from build123d import *

# Parameters (mm, degrees)
F3_DEPTH = 12.7
F5_DEPTH = 12.7


with BuildPart() as f1:
    # F0 (on Front) → F1 (revolve)
    with BuildSketch(Plane.XZ):
        with BuildLine():
            ThreePointArc((17.4752, 17.537158), (8.874046, 19.85641), (0, 20.6375))
            ThreePointArc((0, 20.6375), (-8.874046, 19.85641), (-17.4752, 17.537158))
            Line((-17.4752, 17.537158), (-17.4752, 0))
            Line((-17.4752, 0), (17.4752, 0))
            Line((17.4752, 0), (17.4752, 17.537158))
        make_face()
    revolve(axis=Axis((-4.40496, 0, 0), (1, 0, 0)))

    # F2 (on face) → F3 (cut)
    with BuildSketch(Plane.YZ.offset(17.4752)):
        Polygon((4.7879, -2.764295), (4.7879, 2.764295), (0, 5.528591), (-4.7879, 2.764295), (-4.7879, -2.764295), (0, -5.528591), align=None)
    extrude(amount=-F3_DEPTH, mode=Mode.SUBTRACT)

    # F4 (on face) → F5 (join)
    with BuildSketch(Plane(origin=(-17.4752, 0, 0), x_dir=(0, -1, 0), z_dir=(-1, 0, 0))):
        Polygon((4.7625, -2.749631), (4.7625, 2.749631), (0, 5.499261), (-4.7625, 2.749631), (-4.7625, -2.749631), (0, -5.499261), align=None)
    extrude(amount=F5_DEPTH)


solid = f1.part
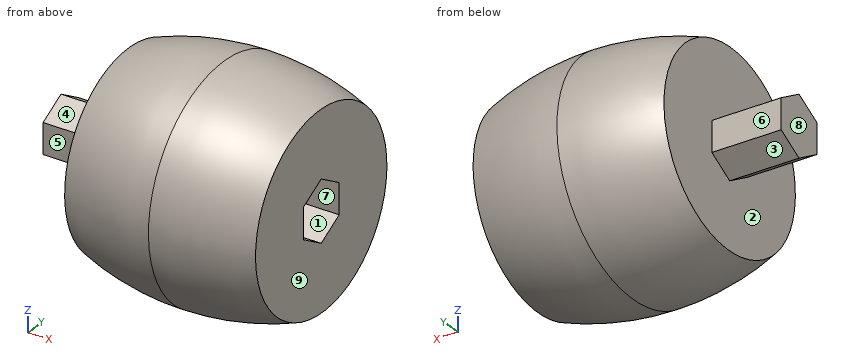
Verification items for the finished model (mm, model axes). Face numbers are marked on the shaded views. A direction names the side the tool comes from. Round coordinates to 2 decimals unless told otherwise and drop trailing zeros. Loops run counter-clockwise (first coordinate to the right, second up) from the corner with the lowest first, then second, coordinate; pieces in that order, holes last. Notation, with made-up numbers: (89.25, -34.75) - (126.25, -34.75) arc R18 ccw to (126.25, -17.75) - close; hole circle Ø10 at (-12.75, -38.75). An arc over 180 degrees is marked (long way). Use a Markdown table: item, result. Add a question column.
1. Gauge pin test, flat ends, axial feed: pin 1 (3 mm diameter, centred on x = 9, z = -0.5, fed in from +Y); pin 2 (3 mm diameter, centred on x = 13.5, z = -1, fed in from -Y); pin 3 (12 mm diameter, centred on y = -3.5, z = -14.5, fed in from -X); pin 4 (12 mm diameter, centred on y = 12, z = -15, fed in from +X). Record the tip position at first contact, or that the pin passes through.
2. Access from +Z, -Z, +X, -X, +Y, -Y to the whole of each face (thin tool, end or side, straight path). Record for the marked faces 5, 6, 7, 8 and 9.
3. Release check for a two-part mould opening along Y. For the marked faces 1, 2, 3 and 4 record: released by +Y, released by -Y, zero draft, split by the parting line, or undercut.
4. Section check A-A, the plane x = -23.5. Record the boundary of the cut face in (y, z), plus the area to 3 significant figures.
5. Thickness scan on probe 1 along X at (y, z) = (-12, 5); probe 2 along X at (y, z) = (0.5, -2); probe 3 along Y at (x, z) = (-10.5, -16). Record the ranges inside material, lowest first. Write a range as [from, to].
Checks:
| question | item | result |
|---|---|---|
| 1 | pin 1 | stops at y = 20.08 |
| 1 | pin 2 | stops at y = -19.18 |
| 1 | pin 3 | stops at x = -17.48 |
| 1 | pin 4 | stops at x = 17.48 |
| 2 | face 5 | +Z, -Z, -X, -Y |
| 2 | face 6 | +Z, -Z, -X, +Y |
| 2 | face 7 | +X |
| 2 | face 8 | +Z, -Z, -X, +Y, -Y |
| 2 | face 9 | +Z, -Z, +X, +Y, -Y |
| 3 | face 1 | undercut |
| 3 | face 2 | zero draft |
| 3 | face 3 | released by +Y |
| 3 | face 4 | released by -Y |
| 4 | outline | (-4.76, -2.75) - (0, -5.5) - (4.76, -2.75) - (4.76, 2.75) - (0, 5.5) - (-4.76, 2.75) - close |
| 4 | area | 78.6 mm^2 |
| 5 | probe 1 | x = [-17.48, 17.48] |
| 5 | probe 2 | x = [-30.18, 4.78] |
| 5 | probe 3 | y = [-11.22, 11.22] |
